from build123d import *

# Parameters (mm, degrees)
F0_W      = 38.1
F0_H      = 76.2
F1_DEPTH  = 177.8
F2_W      = 76.2
F2_H      = 25.4
F3_DEPTH  = 25.4
F5_DEPTH  = 25.4
F7_DEPTH  = 25.4
F9_DEPTH  = 228.6
F11_DEPTH = 228.6
F12_W     = 38.1
F12_H     = 76.2
F13_DEPTH = 25.4
F14_W     = 25.4
F14_H     = 25.4
F15_DEPTH = 228.6
F16_W     = 76.2
F16_H     = 50.8
F17_DEPTH = 38.1
F19_DEPTH = 228.6
F20_W     = 38.1
F20_H     = 76.2
F20_W_2   = 25.4
F20_H_2   = 25.4
F21_DEPTH = 38.1


with BuildPart() as f1:
    # F0 (on Top) → F1 (new body)
    with BuildSketch(Plane.XY):
        Rectangle(F0_W, F0_H)
    extrude(amount=F1_DEPTH)

    # F2 (on face) → F3 (join)
    with BuildSketch(Plane(origin=(-19.05, 0, 0), x_dir=(0, -1, 0), z_dir=(-1, 0, 0))):
        with Locations((0, 127)):
            Rectangle(F2_W, F2_H)
    extrude(amount=F3_DEPTH)

    # F4 (on face) → F5 (join)
    with BuildSketch(Plane.XZ.offset(38.1)):
        Polygon((-44.45, 139.7), (-44.45, 114.3), (-19.05, 114.3), (19.05, 114.3), (19.05, 139.7), (-19.05, 139.7), align=None)
    extrude(amount=F5_DEPTH)

    # F6 (on face) → F7 (join)
    with BuildSketch(Plane(origin=(0, 38.1, 0), x_dir=(-1, 0, 0), z_dir=(0, 1, 0))):
        Polygon((44.45, 114.3), (44.45, 139.7), (19.05, 139.7), (-19.05, 139.7), (-19.05, 114.3), (19.05, 114.3), align=None)
    extrude(amount=F7_DEPTH)

    # F8 (on face) → F9 (cut)
    with BuildSketch(Plane.YZ.offset(19.05)):
        Polygon((-38.1, 114.3), (-63.5, 137.16), (-63.5, 114.3), align=None)
        Polygon((63.5, 137.16), (38.1, 114.3), (63.5, 114.3), align=None)
    extrude(amount=-F9_DEPTH, mode=Mode.SUBTRACT)

    # F10 (on face) → F11 (cut)
    with BuildSketch(Plane.XZ.offset(63.5)):
        Polygon((-19.05, 114.3), (-44.45, 137.16), (-44.45, 114.3), align=None)
    extrude(amount=-F11_DEPTH, mode=Mode.SUBTRACT)

    # F12 (on face) → F13 (join)
    with BuildSketch(Plane.XY.offset(177.8)):
        Rectangle(F12_W, F12_H)
    extrude(amount=F13_DEPTH)

    # F14 (on face) → F15 (cut)
    with BuildSketch(Plane.XY.offset(203.2)):
        Rectangle(F14_W, F14_H)
    extrude(amount=-F15_DEPTH, mode=Mode.SUBTRACT)

    # F16 (on face) → F17 (join)
    with BuildSketch(Plane.YZ.offset(19.05)):
        with Locations((0, 25.4)):
            Rectangle(F16_W, F16_H)
    extrude(amount=F17_DEPTH)

    # F18 (on face) → F19 (cut)
    with BuildSketch(Plane.XZ.offset(38.1)):
        with BuildLine():
            Line((38.1, 50.8), (19.05, 50.8))
            ThreePointArc((19.05, 50.8), (28.575, 49.5901663726), (38.1, 50.8))
        make_face()
    extrude(amount=-F19_DEPTH, mode=Mode.SUBTRACT)

    # F20 (on face) → F21 (cut)
    with BuildSketch(Plane.XY.offset(203.2)):
        Rectangle(F20_W, F20_H)
        Rectangle(F20_W_2, F20_H_2, mode=Mode.SUBTRACT)
    extrude(amount=-F21_DEPTH, mode=Mode.SUBTRACT)


solid = f1.part
For this review, take the finished solid that the model builds, in its own axes (mm). A direction names the side the tool comes from. Round coordinates to 2 decimals unless told otherwise and drop trailing zeros. Order: outer loops, then holes, each group sorted by start corner. A loop starts at its lowest first (then second) coordinate and runs counter-clockwise, first axis right, second up. Notation, with made-up numbers: M 35.25,-18.75 L 56.25,-18.75 A21 ccw 56.25,-0.75 Z; hole C -1,19.25 d6. An arc over 180 degrees is marked long. Write each question's results on one line, items separated by ' | '. Start each with the question number.
1. Add section A-A (x = 8). State the section outline as (y, z) points, then the cut area to 3 significant figures.
2. To check wall thickness, follow L1, parallel to Y at x = -9, z = 36; L2, parallel to X at y = 1.5, z = 35; L3, parallel to Z at x = 50, y = -33.5. State the ranges of each line that lie inside material, in increasing order. Write a range as [from, to].
3. Add section C-C (z = 28). State the section outline as (x, y) points.
4. Draft analysis for pull direction X (two halves, no side actions). For faces 1 (the face through (0, -12.7, 84)), 2 (the face through (0, 38.1, 152)), 3 (the face through (57.15, -1, 26)), state which applies: pulls with the +X half, pulls with the -X half, needs draft (parallel to the pull), parting line crosses it, or undercut.
5. Tool access review of faces 4 (the face through (10, -38.1, 44)), 5 (the face through (12.7, 0, 84)), 6 (the face through (47, -1, 50.8)): name each direction out of +Z, -Z, +X, -X, +Y, -Y from which nothing blocks a thin tool from reaching the whole face with its end or side.
6. Add section D-D (x = -15.5). State the section outline as (y, z) points, then the cut area to 3 significant figures.
7. Clearance check with flat-ended pins moving along their axes: pin 1 Ø1.5 at (x, z) = (11.5, 65.5) entering from +Y; pin 2 Ø8 at (y, z) = (16.5, 18.5) entering from -X; pin 3 Ø20.5 at (x, z) = (-3.5, 75.5) entering from -Y. State where each tip first meets the part, or that it passes through.
8. Add section B-B (y = 8). State the section outline as (x, z) points (3 decimals).
Output values:
1) outline: M -63.5,137.16 L -38.1,114.3 L -38.1,0 L -12.7,0 L -12.7,165.1 L -38.1,165.1 L -38.1,139.7 L -63.5,139.7 Z; M 12.7,0 L 38.1,0 L 38.1,114.3 L 63.5,137.16 L 63.5,139.7 L 38.1,139.7 L 38.1,165.1 L 12.7,165.1 Z | area: 9,100 mm^2
2) L1: [-38.1, -12.7], [12.7, 38.1] | L2: [-19.05, -12.7], [12.7, 57.15] | L3: [0, 50.8]
3) outline: M -19.05,-38.1 L 57.15,-38.1 L 57.15,38.1 L -19.05,38.1 Z; hole M -12.7,-12.7 L 12.7,-12.7 L 12.7,12.7 L -12.7,12.7 Z
4) face 1: undercut | face 2: needs draft | face 3: pulls with the +X half
5) face 4: -Z, +X, -X, -Y | face 5: +Z, -Z | face 6: +Z, +X, +Y, -Y
6) outline: M -63.5,137.16 L -38.1,114.3 L -38.1,0 L 38.1,0 L 38.1,114.3 L 63.5,137.16 L 63.5,139.7 L 38.1,139.7 L 38.1,165.1 L -38.1,165.1 L -38.1,139.7 L -63.5,139.7 Z | area: 13,300 mm^2
7) pin 1: y = 38.1 | pin 2: x = -19.05 | pin 3: y = -38.1
8) outline: M -44.45,137.16 L -19.05,114.3 L -19.05,0 L -12.7,0 L -12.7,165.1 L -19.05,165.1 L -19.05,139.7 L -44.45,139.7 Z; M 12.7,0 L 57.15,0 L 57.15,50.8 L 38.1,50.8 A38.1 cw 19.05,50.8 L 19.05,165.1 L 12.7,165.1 Z
